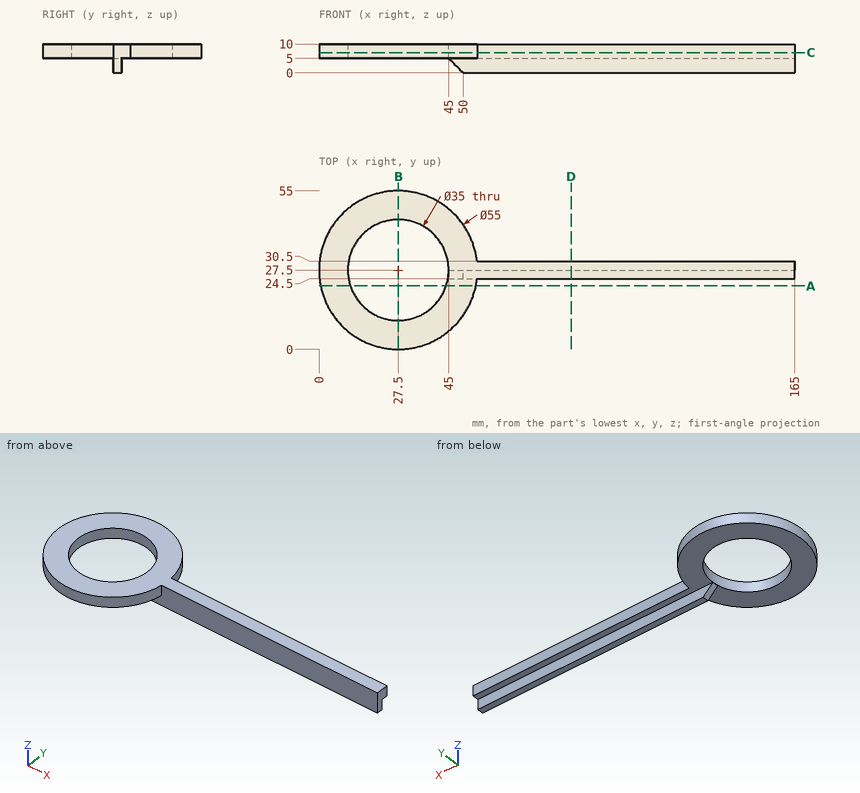
Source: three-view drawing plus pictorial views. Frame: mm from the lowest corner of the part. Round coordinates to 2 decimals unless told otherwise and drop trailing zeros. Order: outer loops, then holes, each group sorted by start corner. A loop starts at its lowest first (then second) coordinate and runs counter-clockwise, first axis right, second up. Notation, with made-up numbers: M 47.25,-35.75 L 62.25,-35.75 A19 ccw 62.25,-27.75 Z; hole C 54.5,16 d3. An arc over 180 degrees is marked long. One line per item, written item: value.
(1) Cut plane C-C (z = 7). Return the cut outline in (x, y).
Result sheet:
outline: M 54.84,24.5 L 165,24.5 L 165,30.5 L 54.84,30.5 A27.5 ccw long Z; hole C 27.5,27.5 d35
(2) Pin query (flat end, axial travel): P1, Ø5.5, axis at x = 95.5, z = 7, coming from the +Y side; P2, Ø6, axis at x = 36.5, z = 5.5, coming from the -Y side; P3, Ø4, axis at y = 43, z = 5.5, coming from the +X side. Return the tip coordinate at first contact, or that it passes through.
Result sheet:
P1: y = 30.5
P2: y = 0.66
P3: x = 51.46
(3) Cut plane A-A (y = 22). Return the cut outline in (x, z), and give its area (3 significant figures).
Result sheet:
outline: M 0.56,5 L 10.89,5 L 10.89,10 L 0.56,10 Z; M 44.11,5 L 54.44,5 L 54.44,10 L 44.11,10 Z
area: 103 mm2
(4) Line query: probe 1 along Z at (x, y) = (40.5, 4); probe 2 along Y at (x, z) = (27.5, 8.75); probe 3 along Y at (x, z) = (61, 3). Output: solid intervals per line, ascending. Write a range as [from, to].
Result sheet:
probe 1: [5, 10]
probe 2: [0, 10], [45, 55]
probe 3: [24.5, 27.5]
(5) Cut plane D-D (x = 87.5). Return the cut outline in (y, z), and give its area (3 significant figures).
Result sheet:
outline: M 24.5,0 L 27.5,0 L 27.5,5 L 30.5,5 L 30.5,10 L 24.5,10 Z
area: 45.0 mm2
(6) Cut plane B-B (x = 27.5). Return the cut outline in (y, z), and give its area (3 significant figures).
Result sheet:
outline: M 0,5 L 10,5 L 10,10 L 0,10 Z; M 45,5 L 55,5 L 55,10 L 45,10 Z
area: 100 mm2
